from build123d import *

# Parameters (mm, degrees)
SKETCH_R     = 13.25
PAD_DEPTH    = 6
FILLET_R     = 1.5
SKETCH001_R  = 2.5
POCKET_DEPTH = 6.001
CHAMFER_SIZE = 2.5


with BuildPart() as part:
    # Sketch → Pad (new body)
    with BuildSketch(Plane.XY):
        Circle(SKETCH_R)
    extrude(amount=PAD_DEPTH)

    # Fillet
    fillet_edges = [part.edges().sort_by_distance(p)[0] for p in [
        (-13.25, 0, 6),
    ]]
    fillet(fillet_edges, radius=FILLET_R)

    # Sketch001 (on Face4 of Fillet) → Pocket (cut, through all)
    with BuildSketch(Plane.XY.offset(6)):
        Circle(SKETCH001_R)
    extrude(amount=-POCKET_DEPTH, mode=Mode.SUBTRACT)

    # Chamfer
    chamfer_edges = [part.edges().sort_by_distance(p)[0] for p in [
        (-2.5, 0, 6),
    ]]
    chamfer(chamfer_edges, length=CHAMFER_SIZE)


solid = part.part
Source: CAD feature listing. Evaluate the final solid. Frame: model axes, mm. Give positions to 0.01 mm unless a question says otherwise; leave off trailing zeros. Write each loop counter-clockwise with the first axis right and the second up, starting at its lowest first coordinate (ties: lowest second). Pieces come first, ordered by that corner, then holes. Notation, with made-up numbers: (27, 70) -> (48, 70) arc R23 ccw to (48, 90) -> close; hole circle Ø1 at (-17.75, -11.75). An arc over 180 degrees is marked (long way). Write item = value, one per line.
Q1. Cut plane A-A on y = 0. Return loops of the section in (x, z).
Here are the results:
outline = (-13.25, 0) -> (-2.5, 0) -> (-2.5, 3.5) -> (-5, 6) -> (-11.75, 6) arc R1.5 ccw to (-13.25, 4.5) -> close; (2.5, 0) -> (13.25, 0) -> (13.25, 4.5) arc R1.5 ccw to (11.75, 6) -> (5, 6) -> (2.5, 3.5) -> close
Q2. Cut plane C-C on z = 2.7. Return loops of the section in (x, y).
Here are the results:
outline = circle Ø26.5 at (0, 0); hole circle Ø5 at (0, 0)
Q3. First-contact query: pin 1 (1 mm diameter, centred on y = 2, z = 1.5, fed in from +X); pin 2 (3 mm diameter, centred on y = -4, z = 4, fed in from -X); pin 3 (2 mm diameter, centred on y = -6.5, z = 1.5, fed in from +X). Flat tips, straight axial feed; report the tip coordinate or a pass-through.
Here are the results:
pin_1 = 13.16
pin_2 = -13.01
pin_3 = 12.05
Q4. Line query: line 1 (Y direction, x = 0, z = 0.9); line 2 (Y direction, x = 1.5, z = 5.25); line 3 (X direction, y = -12, z = 1.55). Output: solid intervals per line, ascending. Write a range as from..to.
Here are the results:
line_1 = -13.25..-2.5, 2.5..13.25
line_2 = -12.96..-3.98, 3.98..12.96
line_3 = -5.62..5.62
